The model under review builds one solid part; all positions refer to its coordinate system, in mm. A direction names the side the tool comes from. Coordinates: 2 decimals unless noted, no trailing zeros. Loops run counter-clockwise (first coordinate to the right, second up) from the corner with the lowest first, then second, coordinate; pieces in that order, holes last. Notation, with made-up numbers: (36.5, -1) - (40.5, -1) arc R22 cw to (40.5, 11) - close; hole circle Ø2 at (-16.5, 30.25). An arc over 180 degrees is marked (long way). One line per item, written item: value. Start each with the question number.
1. Mouldability with a two-part tool opening along Y and no side actions: class faces 1 (the face through (38.1, 82, 0)), 2 (the face through (-1, 82, -2.54)), 3 (the face through (45.33, 3.13, -5.95)), 4 (the face through (1, 166.37, -1)) as +Y half, -Y half, draft (parallel to the pull), parting line (faces both ways), or undercut.
2. To check wall thickness, follow line 1 (Y direction, x = -3, z = 31.5); line 2 (X direction, y = 12.5, z = 0); line 3 (Z direction, x = -35.5, y = 71.5). State the ranges of each line that lie inside material, in increasing order.
3. We need section A-A, the plane z = 17. Give the boundary of the cut face in (x, y), then the cut area to 3 significant figures.
4. We need section D-D, the plane z = -39.5. Give the boundary of the cut face in (x, y).
5. We need section C-C, the plane z = 0. Give the boundary of the cut face in (x, y), then the cut area to 3 significant figures.
6. We need section B-B, the plane x = 0. Give the boundary of the cut face in (y, z).
7. Insertion check: P1, Ø5, axis at x = 23.5, y = 73.5, coming from the +Z side; P2, Ø8, axis at x = -19, z = -26.5, coming from the -Y side; P3, Ø6, axis at x = 27.5, y = 102, coming from the -Z side; P4, Ø5.5, axis at y = 120.5, z = -0.5, coming from the +X side. Each pin has a flat end and moves straight along its axis. Give the tip position at first contact, or say it passes through.
8. For faces 5 (the face through (-38.1, 82, 0)), 6 (the face through (45.33, 163.15, -5.95)), 7 (the face through (-1, 82, 2.54)), list the 3-axis set-ups (+Z, -Z, +X, -X, +Y, -Y) from which the entire face can be reached by the end or side of a thin tool; tool diameter is ignored.
from build123d import *

# Parameters (mm, degrees)
SKETCH1_R           = 45.72
BOSS_EXTRUDE1_DEPTH = 6.35
SKETCH2_W           = 76.2
SKETCH2_H           = 5.08
BOSS_EXTRUDE4_DEPTH = 153.67
SKETCH4_R           = 45.72
BOSS_EXTRUDE5_DEPTH = 6.35


with BuildPart() as part:
    # Sketch1 → Boss-Extrude1 (new body)
    with BuildSketch(Plane(origin=(0, 0, 0), x_dir=(1, 0, 0), z_dir=(0, 1, 0))):
        with Locations(Location((0, 0, 0), (0, 0, 270))):
            Circle(SKETCH1_R)
    extrude(amount=BOSS_EXTRUDE1_DEPTH)

    # Sketch2 → Boss-Extrude4 (add)
    with BuildSketch(Plane(origin=(0, 6.35, 0), x_dir=(1, 0, 0), z_dir=(0, 1, 0))):
        Rectangle(SKETCH2_W, SKETCH2_H)
    extrude(amount=BOSS_EXTRUDE4_DEPTH)

    # Sketch4 → Boss-Extrude5 (add)
    with BuildSketch(Plane(origin=(0, 160.02, 0), x_dir=(1, 0, 0), z_dir=(0, 1, 0))):
        with Locations(Location((0, 0, 0), (0, 0, 270))):
            Circle(SKETCH4_R)
    extrude(amount=BOSS_EXTRUDE5_DEPTH)


solid = part.part
Findings below:
1. face 1: undercut
1. face 2: undercut
1. face 3: draft
1. face 4: +Y half
2. line 1: 0 to 6.35, 160.02 to 166.37
2. line 2: -38.1 to 38.1
2. line 3: -2.54 to 2.54
3. outline: (-42.44, 0) - (42.44, 0) - (42.44, 6.35) - (-42.44, 6.35) - close; (-42.44, 160.02) - (42.44, 160.02) - (42.44, 166.37) - (-42.44, 166.37) - close
3. area: 1,080 mm2
4. outline: (-23.02, 0) - (23.02, 0) - (23.02, 6.35) - (-23.02, 6.35) - close; (-23.02, 160.02) - (23.02, 160.02) - (23.02, 166.37) - (-23.02, 166.37) - close
5. outline: (-45.72, 0) - (45.72, 0) - (45.72, 6.35) - (38.1, 6.35) - (38.1, 160.02) - (45.72, 160.02) - (45.72, 166.37) - (-45.72, 166.37) - (-45.72, 160.02) - (-38.1, 160.02) - (-38.1, 6.35) - (-45.72, 6.35) - close
5. area: 12,900 mm2
6. outline: (0, -45.72) - (6.35, -45.72) - (6.35, -2.54) - (160.02, -2.54) - (160.02, -45.72) - (166.37, -45.72) - (166.37, 45.72) - (160.02, 45.72) - (160.02, 2.54) - (6.35, 2.54) - (6.35, 45.72) - (0, 45.72) - close
7. P1: z = 2.54
7. P2: y = 0
7. P3: z = -2.54
7. P4: x = 38.1
8. face 5: +Z, -Z, -X
8. face 6: +Y, -Y
8. face 7: +Z, +X, -X
